CAD build for the part. Positions are in the model's coordinates, mm. Face numbers are marked on the shaded views. Round coordinates to 2 decimals unless told otherwise and drop trailing zeros.
from build123d import *

# Parameters (mm, degrees)
F0_R     = 38.1
F2_DEPTH = 2.54
F1_R     = 35.56
F1_R_2   = 1.651
F3_DEPTH = 10.16
F4_R     = 2.4379748878
F4_R_2   = 2.3255862578
F4_R_3   = 2.3096296398
F5_DEPTH = 2.541
F6_R     = 33.02
F6_R_2   = 32.2280056546
F7_DEPTH = 10.16


with BuildPart() as f2:
    # F0 (on Top) → F2 (new body)
    with BuildSketch(Plane.XY):
        Circle(F0_R)
    extrude(amount=-F2_DEPTH)

    # F1 (on Top) → F3 (join)
    with BuildSketch(Plane.XY):
        Circle(F1_R)
        with BuildLine():
            ThreePointArc((31.0887399015, 11.1270234717), (32.5336025637, 5.6466896698), (33.02, 0))
            ThreePointArc((33.02, 0), (33.012710709, -0.6937806881), (32.9908460543, -1.3872550667))
            ThreePointArc((32.9908460543, -1.3872550667), (32.3733882594, -6.5026250548), (30.9676692654, -11.4596623105))
            ThreePointArc((30.9676692654, -11.4596623105), (28.197005304, -17.1828196722), (24.3807439254, -22.2688061118))
            ThreePointArc((24.3807439254, -22.2688061118), (20.6196473654, -25.7905126457), (16.3564820127, -28.6842447376))
            ThreePointArc((16.3564820127, -28.6842447376), (10.5552556409, -31.2874891667), (4.3626207519, -32.730535287))
            ThreePointArc((4.3626207519, -32.730535287), (-0.7822556928, -33.01073274), (-5.9080849557, -32.4871502622))
            ThreePointArc((-5.9080849557, -32.4871502622), (-12.0254154451, -30.7523947583), (-17.6968211565, -27.877283242))
            ThreePointArc((-17.6968211565, -27.877283242), (-21.8181326185, -24.7848641118), (-25.4081933124, -21.0889571246))
            ThreePointArc((-25.4081933124, -21.0889571246), (-28.9792609968, -15.8279130678), (-31.4757237675, -9.9799405466))
            ThreePointArc((-31.4757237675, -9.9799405466), (-32.6450628105, -4.9618821127), (-33.0195256375, 0.1769934293))
            ThreePointArc((-33.0195256375, 0.1769934293), (-32.3733882594, 6.5026250548), (-30.526785414, 12.5871272453))
            ThreePointArc((-30.526785414, 12.5871272453), (-28.197005304, 17.1828196722), (-25.1806549457, 21.3601267905))
            ThreePointArc((-25.1806549457, 21.3601267905), (-20.6196473654, 25.7905126457), (-15.2940248979, 29.2645383087))
            ThreePointArc((-15.2940248979, 29.2645383087), (-10.5552556409, 31.2874891667), (-5.559475953, 32.5486194351))
            ThreePointArc((-5.559475953, 32.5486194351), (0.7822556928, 33.01073274), (7.0949798421, 32.2487466584))
            ThreePointArc((7.0949798421, 32.2487466584), (12.0254154451, 30.7523947583), (16.6630436248, 28.5072513084))
            ThreePointArc((16.6630436248, 28.5072513084), (21.8181326185, 24.7848641118), (26.1641646621, 20.1434080418))
            ThreePointArc((26.1641646621, 20.1434080418), (28.9792609968, 15.8279130678), (31.0887399015, 11.1270234717))
        make_face(mode=Mode.SUBTRACT)
        Polygon((2.6006015495, 20.4516352474), (5.0752879427, 23.8023692852), (-3.0012168531, 23.8023692852), (-5.4759032463, 20.4516352474), align=None)
        Polygon((12.5755624743, 17.032619561), (17.6111808492, 10.7181538433), (21.7738319382, 10.8725146132), (16.7382135634, 17.1869803309), align=None)
        Polygon((21.157373157, 0.787693943), (19.3601817668, -7.0863160152), (22.0762363791, -10.2445653214), (23.8734277693, -2.3705553631), align=None)
        Polygon((13.8072503208, -16.05038128), (6.5305709383, -19.5546453798), (5.7547845533, -23.6472786179), (13.0314639358, -20.1430145181), align=None)
        Polygon((-3.9400136236, -20.8021920311), (-11.2166930061, -17.2979279313), (-14.9001374173, -19.2431087986), (-7.6234580348, -22.7473728984), align=None)
        Polygon((-18.7203669478, -9.8895278954), (-20.5175583381, -2.0155179371), (-24.3349520053, -0.348485566), (-22.537760615, -8.2224955243), align=None)
        Polygon((-19.4039021344, 8.4701524552), (-14.3682837595, 14.7846181728), (-15.4450513907, 18.8085544056), (-20.4806697656, 12.4940886879), align=None)
        Polygon((2.3585940213, 10.6214470988), (4.8124587489, 13.8745305248), (-3.2640460469, 13.8745305248), (-5.7179107745, 10.6214470988), align=None)
        Polygon((10.8304421112, 1.0390514452), (14.6825942043, -0.2894545314), (12.1868169672, 7.3917579835), (8.3346648742, 8.7202639601), align=None)
        Polygon((4.3349873167, -9.9792779897), (4.2618835124, -14.0534232634), (10.7959131473, -9.3061728544), (10.8690169516, -5.2320275806), align=None)
        Polygon((-8.1512726087, -7.206584426), (-12.0486053375, -8.3960387037), (-5.5145757026, -13.1432891127), (-1.6172429738, -11.953834835), align=None)
        Polygon((-9.3727508404, 5.5253638716), (-11.708331128, 8.8643859737), (-14.2041083651, 1.1831734587), (-11.8685280775, -2.1558486433), align=None)
        Polygon((0, -4.8615827019), (4.2102541225, 2.430791351), (-4.2102541225, 2.430791351), align=None)
        Circle(F1_R_2, mode=Mode.SUBTRACT)
    extrude(amount=F3_DEPTH)

    # F4 (on face) → F5 (cut, through all)
    with BuildSketch(Plane.XY):
        with Locations((-7.6389224268, 28.7674851716)):
            Circle(F4_R)
        with Locations((-24.3431371066, 17.1269674708)):
            Circle(F4_R)
        with Locations((-29.6569273904, -2.5274486545)):
            Circle(F4_R)
        with Locations((-21.0939117481, -20.999243465)):
            Circle(F4_R)
        with Locations((-2.6608203662, -29.6452588776)):
            Circle(F4_R)
        with Locations((17.0172984368, -24.419928191)):
            Circle(F4_R)
        with Locations((28.732834175, -7.7682417066)):
            Circle(F4_R)
        with Locations((27.0039574729, 12.5182914067)):
            Circle(F4_R)
        with Locations((12.6396289536, 26.9473768455)):
            Circle(F4_R)
        with Locations((-11.462688446, 20.8468269557)):
            Circle(F4_R_2)
        with Locations((-23.4455749715, 4.0358933071)):
            Circle(F4_R_2)
        with Locations((-17.7734653408, -15.8141503189)):
            Circle(F4_R_2)
        with Locations((1.2824262041, -23.7558162049)):
            Circle(F4_R_2)
        with Locations((19.3726246606, -13.8088679583)):
            Circle(F4_R_2)
        with Locations((22.8748416182, 6.5364395105)):
            Circle(F4_R_2)
        with Locations((9.1518362755, 21.9596747088)):
            Circle(F4_R_2)
        with Locations((-9.2776790261, 12.2433528304)):
            Circle(F4_R_3)
        with Locations((-14.5110809781, -5.0401930012)):
            Circle(F4_R_3)
        with Locations((0.3093377682, -15.358363415)):
            Circle(F4_R_3)
        with Locations((14.7022622328, -4.4517976009)):
            Circle(F4_R_3)
        with Locations((8.7771600032, 12.6070011866)):
            Circle(F4_R_3)
    extrude(amount=-F5_DEPTH, mode=Mode.SUBTRACT)

    # F6 (on face) → F7 (join, through all)
    with BuildSketch(Plane.XY):
        Circle(F6_R)
        Circle(F6_R_2, mode=Mode.SUBTRACT)
    extrude(amount=F7_DEPTH)


solid = f2.part
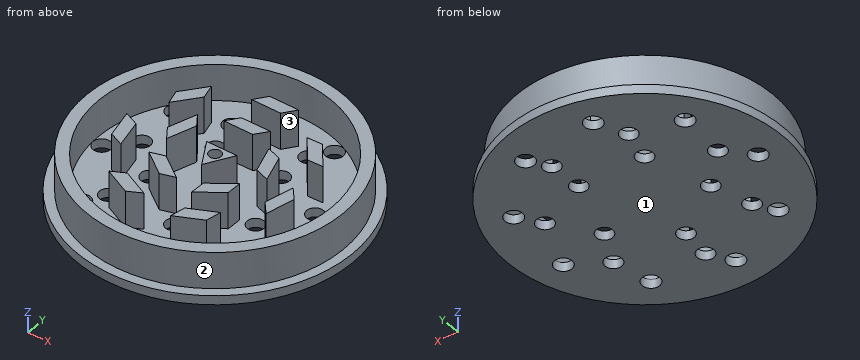
Item 1: Wall check: L1, parallel to Y at x = -18, z = 9.5; L2, parallel to Y at x = 11.5, z = 4.25; L3, parallel to X at y = -3.5, z = 8.25. Give the ranges that are in metal, low to high.
Verdict:
L1: y = -30.67 to -26.73, 10.23 to 15.6, 26.73 to 30.67
L2: y = -33.65 to -30.11, -20.88 to -17.16, 0.81 to 7.63, 30.11 to 33.65
L3: x = -35.39 to -32.04, -23.62 to -20.18, -0.79 to 0.79, 20.18 to 23.62, 32.04 to 35.39
Item 2: Flat gauge pins, fed straight in: P1, Ø4, axis at x = -24.34, y = 17.13, coming from the +Z side; P2, Ø2.5, axis at x = 2.5, z = 3, coming from the +Y side; P3, Ø1.7, axis at x = -0.5, y = 0, coming from the +Z side; P4, Ø4, axis at x = -2.5, z = 7.5, coming from the -Y side. Where does each tip first touch, or does it go through?
Verdict:
P1: passes through
P2: stops at y = 35.54
P3: stops at z = 0
P4: stops at y = -35.56
Item 3: Cut at A-A (z = -1.5). State how many separate pieces and enclosed holes the cut face has, plus the area to 3 significant figures.
Verdict:
separate pieces: 1
enclosed holes: 21
area: 4,190 mm2
Item 4: Mould opens along Y. For the marked faces 1, 2 and 3 say: released by +Y, released by -Y, zero draft, split by the parting line, or undercut.
Verdict:
face 1: zero draft
face 2: split by the parting line
face 3: undercut
